Model file for the job. Use its own axes, mm. Face numbers are marked on the shaded views. A direction names the side the tool comes from. Round coordinates to 2 decimals unless told otherwise and drop trailing zeros. Loops run counter-clockwise (first coordinate to the right, second up) from the corner with the lowest first, then second, coordinate; pieces in that order, holes last. Notation, with made-up numbers: M 32.5,-25 L 84.5,-25 A13 cw 84.5,-10 Z; hole C 50.5,87.5 d1. An arc over 180 degrees is marked long. Use a Markdown table: item, result. Add a question column.
Item 1: Wall check: L1, parallel to Z at x = 0.95, y = 7.5; L2, parallel to X at y = 1.4, z = 5. Give the ranges that are in metal, low to high. Write a range as from..to.
Item 2: Saw through at B-B on x = 6.75. Write the cut outline in (y, z).
Item 3: Pin check, flat tips, straight feed: P1, Ø1, axis at y = 5, z = 23, coming from the +X side; P2, Ø2, axis at y = 7.5, z = 25, coming from the +X side; P3, Ø6.5, axis at x = 9, z = 16.5, coming from the +Y side. Stop position of each tip, or through.
Item 4: Saw through at A-A on z = 25. Write the cut outline in (x, y), then the cut area to 3 significant figures.
Item 5: Saw through at D-D on z = 3. Write the cut outline in (x, y), then the cut area to 3 significant figures.
Item 6: Saw through at C-C on y = 7.5. Write the cut outline in (x, z).
Item 7: Tool access for the marked faces 1 and 2: list every direction of +Z, -Z, +X, -X, +Y, -Y with a clear straight run to the whole face (end or side of a thin tool).
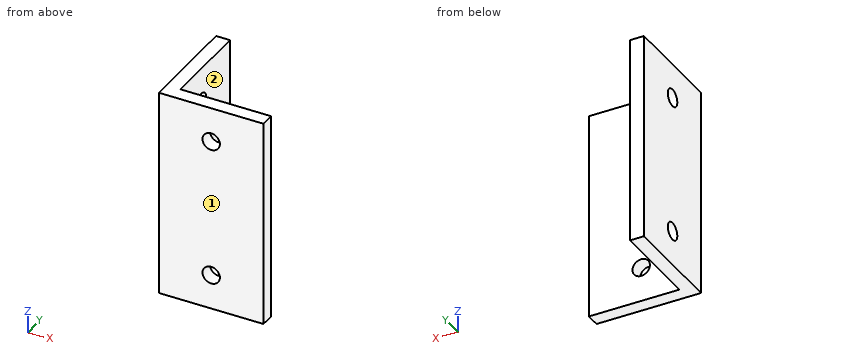
```python
from build123d import *

# Parameters (mm, degrees)
EXTRUDE_1_DEPTH          = 30
M3X0_5_1_D               = 2.5
M3X0_5_1_DEPTH           = 8.5
M3X0_5_1_TIP             = 0.751075774
M3X0_5_1_ON_FACE_2_D     = 2.5
M3X0_5_1_ON_FACE_2_DEPTH = 8.5
M3X0_5_1_ON_FACE_2_TIP   = 0.751075774


with BuildPart() as part:
    # ｽｹｯﾁ1 → ﾎﾞｽ - 押し出し1 (new body)
    with BuildSketch(Plane.XY):
        Polygon((0, 0), (0, 15), (2, 15), (2, 2), (15, 2), (15, 0), align=None)
    extrude(amount=EXTRUDE_1_DEPTH)

    # M3x0.5 ねじ穴1
    with Locations(Plane(origin=(7.5, 0, 5), x_dir=(0, 0, -1), z_dir=(0, -1, 0))):
        with Locations((0, 0), (-20, 0)):
            Hole(M3X0_5_1_D / 2, depth=M3X0_5_1_DEPTH)
            with Locations((0, 0, -(M3X0_5_1_DEPTH + M3X0_5_1_TIP / 2))):  # 118° drill point
                Cone(0, M3X0_5_1_D / 2, M3X0_5_1_TIP, mode=Mode.SUBTRACT)

    # M3x0.5 ねじ穴1 on face 2
    with Locations(Plane(origin=(0, 7.5, 25), x_dir=(0, 0, -1), z_dir=(-1, 0, 0))):
        with Locations((0, 0), (20, 0)):
            Hole(M3X0_5_1_ON_FACE_2_D / 2, depth=M3X0_5_1_ON_FACE_2_DEPTH)
            with Locations((0, 0, -(M3X0_5_1_ON_FACE_2_DEPTH + M3X0_5_1_ON_FACE_2_TIP / 2))):  # 118° drill point
                Cone(0, M3X0_5_1_ON_FACE_2_D / 2, M3X0_5_1_ON_FACE_2_TIP, mode=Mode.SUBTRACT)


solid = part.part
```
Entries:
| question | item | result |
|---|---|---|
| 1 | L1 | 0..3.75, 6.25..23.75, 26.25..30 |
| 1 | L2 | 0..6.25, 8.75..15 |
| 2 | outline | M 0,0 L 2,0 L 2,4 L 0,4 Z; M 0,6 L 2,6 L 2,24 L 0,24 Z; M 0,26 L 2,26 L 2,30 L 0,30 Z |
| 3 | P1 | x = 2 |
| 3 | P2 | through |
| 3 | P3 | y = 2 |
| 4 | outline | M 0,0 L 6.25,0 L 6.25,2 L 2,2 L 2,6.25 L 0,6.25 Z; M 0,8.75 L 2,8.75 L 2,15 L 0,15 Z; M 8.75,0 L 15,0 L 15,2 L 8.75,2 Z |
| 4 | area | 46.0 mm2 |
| 5 | outline | M 0,0 L 15,0 L 15,2 L 2,2 L 2,15 L 0,15 Z |
| 5 | area | 56.0 mm2 |
| 6 | outline | M 0,0 L 2,0 L 2,3.75 L 0,3.75 Z; M 0,6.25 L 2,6.25 L 2,23.75 L 0,23.75 Z; M 0,26.25 L 2,26.25 L 2,30 L 0,30 Z |
| 7 | face 1 | +Z, -Z, +X, -X, -Y |
| 7 | face 2 | +Z, -Z, +X, +Y |
